Read the model definition and answer for the solid it produces. Units are mm, in the model's axes. A direction names the side the tool comes from. Coordinates: 2 decimals unless noted, no trailing zeros. Order: outer loops, then holes, each group sorted by start corner. A loop starts at its lowest first (then second) coordinate and runs counter-clockwise, first axis right, second up. Notation, with made-up numbers: (83.5, 57.25) -> (91.5, 57.25) arc R24 ccw to (91.5, 71.25) -> close; hole circle Ø6 at (-31.75, -34.5). An arc over 180 degrees is marked (long way). Use CSV: the item, a comma, the result in double quotes.
```python
from build123d import *

# Parameters (mm, degrees)
F0_W     = 25
F0_H     = 50
F1_DEPTH = 50
F2_W     = 10
F2_H     = 30
F3_DEPTH = 25
F5_R     = 5
F6_DEPTH = 25


with BuildPart() as f1:
    # F0 (on Right) → F1 (new body, symmetric)
    with BuildSketch(Plane.YZ):
        Rectangle(F0_W, F0_H)
    extrude(amount=F1_DEPTH, both=True)

    # F2 (on face) → F3 (join)
    with BuildSketch(Plane.YZ.offset(50)):
        Rectangle(F2_W, F2_H)
    extrude(amount=F3_DEPTH)

    # F4: F1 across plane


with BuildPart() as f1_1:
    add(f1.part)
    add(f1.part.mirror(Plane.YZ))

    # F5 (on face) → F6 (cut)
    with BuildSketch(Plane.XY.offset(25)):
        with Locations((-25, 0)):
            Circle(F5_R)
        with Locations((25, 0)):
            Circle(F5_R)
    extrude(amount=-F6_DEPTH, mode=Mode.SUBTRACT)


solid = f1_1.part
```
Item 1: Find section C-C, the plane x = 25. Give the vertices of the cut face in (y, z).
Return value:
outline,"(-12.5, -25) -> (12.5, -25) -> (12.5, 25) -> (5, 25) -> (5, 0) -> (-5, 0) -> (-5, 25) -> (-12.5, 25) -> close"
Item 2: Find section B-B, the plane y = 0. Give the vertices of the cut face in (x, z).
Return value:
outline,"(-75, -15) -> (-50, -15) -> (-50, -25) -> (50, -25) -> (50, -15) -> (75, -15) -> (75, 15) -> (50, 15) -> (50, 25) -> (30, 25) -> (30, 0) -> (20, 0) -> (20, 25) -> (-20, 25) -> (-20, 0) -> (-30, 0) -> (-30, 25) -> (-50, 25) -> (-50, 15) -> (-75, 15) -> close"
Item 3: Find section D-D, the plane z = -6.5. Give the vertices of the cut face in (x, y).
Return value:
outline,"(-75, -5) -> (-50, -5) -> (-50, -12.5) -> (50, -12.5) -> (50, -5) -> (75, -5) -> (75, 5) -> (50, 5) -> (50, 12.5) -> (-50, 12.5) -> (-50, 5) -> (-75, 5) -> close"
Item 4: Straight lines are drawn through the part: line 1 along Y through (x, z) = (-25, 19.25); line 2 along Y through (x, z) = (-60, 9); line 3 along X through (y, z) = (-5.75, -9). For each, find the intervals that lie inside material, in ascending order.
Return value:
line 1,"y = -12.5 to -5, 5 to 12.5"
line 2,"y = -5 to 5"
line 3,"x = -50 to 50"
Item 5: A tool of negligible diameter and unlimited length cuts with its end or side. For faces 1 (the flat face through (-62, 0, -15)), 2 (the flat face through (62, -5, 0)), 3 (the cylindrical face through (20, 0, 13)), 4 (the flat face through (-62, -5, 0)), 5 (the flat face through (62, 5, 0)), from which of +Z, -Z, +X, -X, +Y, -Y can it reach the whole face along a straight path? Write none if from no direction.
Return value:
face 1,"-Z, -X, +Y, -Y"
face 2,"+Z, -Z, +X, -Y"
face 3,"+Z"
face 4,"+Z, -Z, -X, -Y"
face 5,"+Z, -Z, +X, +Y"
Item 6: The mould has two halves that part along Y. Classify faces 6 (the flat face through (-62, 0, 15)), 7 (the flat face through (-25, 0, 0)), 8 (the flat face through (-62, 5, 0)): +Y half, -Y half, draft (parallel to the pull), parting line (faces both ways), or undercut.
Return value:
face 6,"draft"
face 7,"undercut"
face 8,"+Y half"
Item 7: Each of these flat-tipped pins is pushed along its axis until it touches: P1, Ø5, axis at x = -64, y = -2, coming from the -Z side; P2, Ø11.5, axis at x = 25, y = 0, coming from the +Z side; P3, Ø1.5, axis at y = -6, z = 16, coming from the -X side; P4, Ø3, axis at x = 65.5, y = -1.5, coming from the +Z side. Where does it stop, or does it pass through?
Return value:
P1,"stops at z = -15"
P2,"stops at z = 25"
P3,"stops at x = -50"
P4,"stops at z = 15"
Item 8: Find section A-A, the plane z = 12. Give the vertices of the cut face in (x, y).
Return value:
outline,"(-75, -5) -> (-50, -5) -> (-50, -12.5) -> (50, -12.5) -> (50, -5) -> (75, -5) -> (75, 5) -> (50, 5) -> (50, 12.5) -> (-50, 12.5) -> (-50, 5) -> (-75, 5) -> close; hole circle Ø10 at (-25, 0); hole circle Ø10 at (25, 0)"
